Autodesk Inventor part; units mm, degrees
sketch "Эскиз2" plane through (0, 0, 0) normal (0, 1, 0) x (-1, 0, 0)
  line L0 (105, 150) -> (-105, 150)
  line L1 (-105, 150) -> (-105, -150)
  line L2 (-105, -150) -> (105, -150)
  line L3 (105, -150) -> (105, 150)
  line L4 (105, 150) -> (-105, -150) construction
  line L5 (-105, 150) -> (105, -150) construction
  point P0 (0, 0)
  dimension "d0" = 300
  dimension "d1" = 210
extrude "Выдавливание1" add sketch "Эскиз2" along normal mid plane 4
sketch "Эскиз3" plane through (0, -2, 0) normal (0, -1, 0) x (1, 0, 0)
  line L0 (105, -150) -> (-105, -150)
  line L1 (20, -150) -> (-20, -150)
  line L2 (-20, -150) -> (-20, -70)
  line L3 (-20, -70) -> (20, -70)
  line L4 (20, -70) -> (20, -150)
  line L5 (-105, 150) -> (-105, -150)
  line L6 (20, -130) -> (-20, -130)
  dimension "d7" = 40
  dimension "d9" = 80
  dimension "d10" = 20
  dimension "d12" = 85
extrude "Выдавливание2" cut sketch "Эскиз3" against normal up to next contours L6 L2 L3 L4
fillet "Сопряжение1" radius 10 4 edges at (20, 0, -130) (-20, 0, -130) (-20, 0, -70) (20, 0, -70)
ref_plane "РабПлоскость1" through (-10, -2, -100) normal (0, 0, 1) x (1, 0, 0)
properties part number "Передняя_фанера"
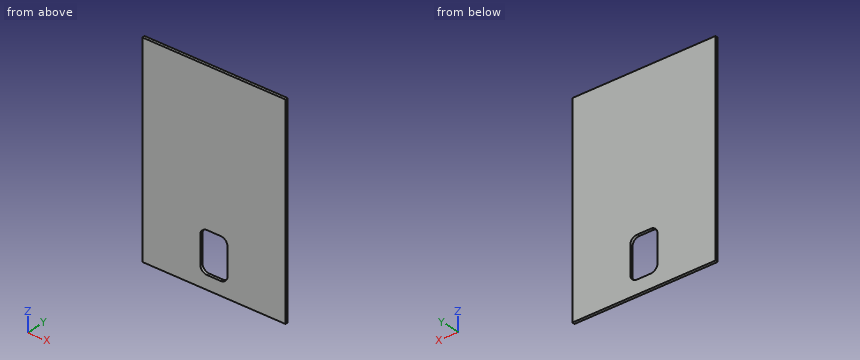
Input: part model. Units: mm. Frame: model coordinates. Coordinates: 2 decimals unless noted, no trailing zeros. Loops run counter-clockwise (first coordinate to the right, second up) from the corner with the lowest first, then second, coordinate; pieces in that order, holes last.
(1) Section C-C on z = -75.5. Return the cut outline in (x, y).
(2) Section A-A on z = -126. Return the cut outline in (x, y).
(3) Section B-B on y = 0.85. Return the cut outline in (x, z), then the cut area to 3 significant figures.
(4) Material intervals for probe 1 along X at (y, z) = (-1.4, -111); probe 2 along Z at (x, y) = (8, 1); probe 3 along Z at (x, y) = (-17.5, -0.6), sorted ascending.
(5) First-contact query: pin 1 Ø6 at (x, z) = (17.5, -119.5) entering from +Y. Flat tip, straight axial feed; report the tip coordinate or a pass-through.
Data:
1. outline: (-105, -2) - (-18.93, -2) - (-18.93, 2) - (-105, 2) - close; (18.93, -2) - (105, -2) - (105, 2) - (18.93, 2) - close
2. outline: (-105, -2) - (-18, -2) - (-18, 2) - (-105, 2) - close; (18, -2) - (105, -2) - (105, 2) - (18, 2) - close
3. outline: (-105, -150) - (105, -150) - (105, 150) - (-105, 150) - close; hole (-20, -120) arc R10 ccw to (-10, -130) - (10, -130) arc R10 ccw to (20, -120) - (20, -80) arc R10 ccw to (10, -70) - (-10, -70) arc R10 ccw to (-20, -80) - close
3. area: 60,700 mm2
4. probe 1: x = -105 to -20, 20 to 105
4. probe 2: z = -150 to -130, -70 to 150
4. probe 3: z = -150 to -126.61, -73.39 to 150
5. pin 1: stops at y = 2
